The listing builds one solid part. Answer for the finished solid, in the listing's coordinates (mm). Give positions to 0.01 mm unless a question says otherwise; leave off trailing zeros. Loops run counter-clockwise (first coordinate to the right, second up) from the corner with the lowest first, then second, coordinate; pieces in that order, holes last.
Item 1: Section C-C, the plane y = 58 is taken. Give the vertices of the cut face in (x, z).
Item 2: Section B-B, the plane z = 5.75 is taken. Give the number of separate pieces and of enclosed holes in the cut face, and give its area (3 significant figures).
Item 3: Consider line 1 along X through (y, z) = (22.25, 4.5); line 2 along Y through (x, z) = (33.5, 7.25); line 3 along X through (y, z) = (35, 4.25). Determine where each line is inside the solid, lowest interval first.
Item 4: Section A-A, the plane y = 113 is taken. Give the vertices of the cut face in (x, z).
Item 5: Each of these flat-tipped pins is pushed along its axis until it touches: pin 1 Ø5 at (x, y) = (-3, 114.5) entering from -Z; pin 2 Ø8 at (x, y) = (171.5, 123.5) entering from +Z; pin 3 Ø4 at (x, z) = (-5.5, 5.5) entering from -Y. Where does it stop, or does it pass through?
from build123d import *

# Parameters (mm, degrees)
SKETCH_1_W          = 164
SKETCH_1_H          = 180
EXTRUDE_1_DEPTH     = 10
SKETCH_2_W          = 4.9
SKETCH_2_H          = 159.9
EXTRUDE_2_DEPTH     = 10
SKETCH_3_R          = 2
CUT_EXTRUDE_1_DEPTH = 10
SKETCH_7_R          = 2.25
SKETCH_7_W          = 30
SKETCH_7_H          = 55
CUT_EXTRUDE_5_DEPTH = 251.551391934


with BuildPart() as part:
    # 草图1 → 凸台-拉伸1 (new body)
    with BuildSketch(Plane.XY):
        with Locations((82, 90)):
            Rectangle(SKETCH_1_W, SKETCH_1_H)
    extrude(amount=EXTRUDE_1_DEPTH)

    # 草图2 → 凸台-拉伸2 (add)
    with BuildSketch(Plane.ZY):
        with Locations((5, 90)):
            Rectangle(SKETCH_2_W, SKETCH_2_H)
    extrude_2 = extrude(amount=EXTRUDE_2_DEPTH)

    # 镜向1: 凸台-拉伸2 across plane
    add(extrude_2.mirror(Plane(origin=(82, 0, 0), x_dir=(0, 0, 1), z_dir=(1, 0, 0))))

    # 草图3 → 切除-拉伸1 (cut)
    with BuildSketch(Plane(origin=(0, 0, 0), x_dir=(-1, 0, 0), z_dir=(0, 0, -1))):
        with Locations((-149.6425573, 145)):
            Circle(SKETCH_3_R)
        with Locations((-130.5, 157.75)):
            Circle(SKETCH_3_R)
        with Locations((-130.5, 132.25)):
            Circle(SKETCH_3_R)
        with Locations((-14.3574427, 145)):
            Circle(SKETCH_3_R)
        with Locations((-33.5, 157.75)):
            Circle(SKETCH_3_R)
        with Locations((-33.5, 132.25)):
            Circle(SKETCH_3_R)
        with Locations(Location((-130.5, 47.75, 0), (0, 0, 180))):
            Circle(SKETCH_3_R)
        with Locations(Location((-130.5, 22.25, 0), (0, 0, 180))):
            Circle(SKETCH_3_R)
        with Locations(Location((-149.6425573, 35, 0), (0, 0, 180))):
            Circle(SKETCH_3_R)
        with Locations(Location((-33.5, 47.75, 0), (0, 0, 180))):
            Circle(SKETCH_3_R)
        with Locations(Location((-33.5, 22.25, 0), (0, 0, 180))):
            Circle(SKETCH_3_R)
        with Locations(Location((-14.3574427, 35, 0), (0, 0, 180))):
            Circle(SKETCH_3_R)
    extrude(amount=-CUT_EXTRUDE_1_DEPTH, mode=Mode.SUBTRACT)

    # 草图7 → 切除-拉伸5 (cut, through all)
    with BuildSketch(Plane.XY.offset(10)):
        with Locations((120, 105)):
            Circle(SKETCH_7_R)
        with Locations((120, 75)):
            Circle(SKETCH_7_R)
        with Locations((100, 105)):
            Circle(SKETCH_7_R)
        with Locations((100, 75)):
            Circle(SKETCH_7_R)
        with Locations((149, 90)):
            Rectangle(SKETCH_7_W, SKETCH_7_H)
    extrude(amount=-CUT_EXTRUDE_5_DEPTH, mode=Mode.SUBTRACT)


solid = part.part
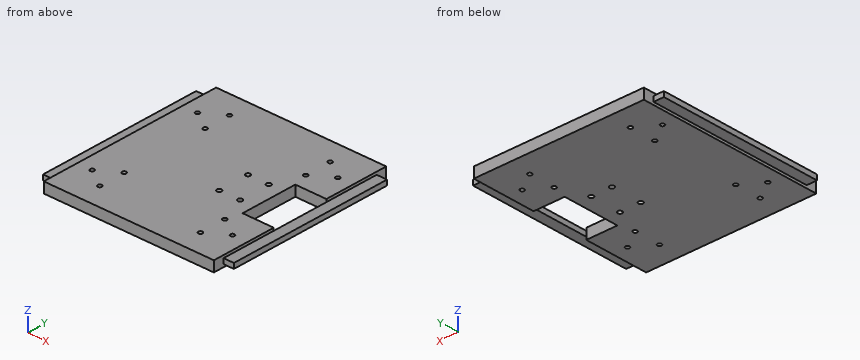
Worked answers:
1. outline: (-10, 2.55) - (0, 2.55) - (0, 0) - (164, 0) - (164, 2.55) - (174, 2.55) - (174, 7.45) - (164, 7.45) - (164, 10) - (0, 10) - (0, 7.45) - (-10, 7.45) - close
2. separate pieces: 1
2. enclosed holes: 17
2. area: 30,900 mm2
3. line 1: x = -10 to 31.5, 35.5 to 128.5, 132.5 to 174
3. line 2: y = 0 to 20.25, 24.25 to 45.75, 49.75 to 130.25, 134.25 to 155.75, 159.75 to 180
3. line 3: x = -10 to 12.36, 16.36 to 147.64, 151.64 to 174
4. outline: (-10, 2.55) - (0, 2.55) - (0, 0) - (134, 0) - (134, 10) - (0, 10) - (0, 7.45) - (-10, 7.45) - close; (164, 2.55) - (174, 2.55) - (174, 7.45) - (164, 7.45) - close
5. pin 1: stops at z = 2.55
5. pin 2: stops at z = 7.45
5. pin 3: stops at y = 10.05
